from build123d import *

# Parameters (mm, degrees)
EXTRUDE_THIN1_DEPTH             = 57.15
M2_5_CLEARANCE_HOLE1_AT_2_COUNT = 2
M2_5_CLEARANCE_HOLE1_AT_2_PITCH = 6.096
CUT_EXTRUDE1_REACH              = 141.7
SKETCH2_R                       = 6.35
CIRPATTERN1_COUNT               = 8
CUT_EXTRUDE2_REACH              = 59.15
SKETCH5_R                       = 3.5
CIRPATTERN2_COUNT               = 4


with BuildPart() as part:
    # Sketch1 → Extrude-Thin1 (new body)
    with BuildSketch(Plane(origin=(0, 0, 0), x_dir=(0, 0, -1), z_dir=(1, 0, 0))):
        Polygon((0, 0), (57.15, 0), (57.15, -139.7), (52.324, -139.7), (52.324, -4.826), (0, -4.826), align=None)
    extrude(amount=EXTRUDE_THIN1_DEPTH)

    # Sketch4 → M2.5 Clearance Hole1 (revolve, cut)
    with BuildSketch(Plane(origin=(17.349679849, 0, -39.800320151), x_dir=(0, 0, 1), z_dir=(1, 0, 0))):
        Polygon((0, 0), (0, 5.89269403), (1.35255, 5.08), (1.35255, 0), align=None)
    m2_5_clearance_hole1 = revolve(axis=Axis((17.349679849, 6.35, -39.800320151), (0, -1, 0)), mode=Mode.SUBTRACT)

    # M2.5 Clearance Hole1 at 2: M2.5 Clearance Hole1 ×2
    with Locations(*[Vector(0.707106781, 0, 0.707106781) * (i * M2_5_CLEARANCE_HOLE1_AT_2_PITCH) for i in range(1, M2_5_CLEARANCE_HOLE1_AT_2_COUNT)]):
        add(m2_5_clearance_hole1, mode=Mode.SUBTRACT)

    # Sketch2 → Cut-Extrude1 (cut, up to next)
    with BuildSketch(Plane(origin=(0, 0, 0), x_dir=(1, 0, 0), z_dir=(0, 1, 0)), mode=Mode.PRIVATE) as cut_extrude1_sk1:
        with Locations((28.575, 28.575)):
            Circle(SKETCH2_R)
    cut_extrude1_tool1 = extrude(cut_extrude1_sk1.sketch, amount=-CUT_EXTRUDE1_REACH, mode=Mode.PRIVATE) & part.part
    add(cut_extrude1_tool1.solids().sort_by_distance((28.575, 0, -28.575))[0], mode=Mode.SUBTRACT)

    # CirPattern1: M2.5 Clearance Hole1 ×8 about axis
    cirpattern1_axis = Axis((28.575, 0, -28.575), (0, 1, 0))
    for i in range(1, CIRPATTERN1_COUNT):
        add(m2_5_clearance_hole1.rotate(cirpattern1_axis, i * 360 / CIRPATTERN1_COUNT), mode=Mode.SUBTRACT)

    # CirPattern1 copy 1 sketch → CirPattern1 copy 1 (revolve, cut)
    with BuildSketch(Plane(origin=(18.796, 0, -28.575), x_dir=(0.707106781, 0, 0.707106781), z_dir=(0.707106781, 0, -0.707106781))):
        Polygon((0, 0), (0, 5.89269403), (1.35255, 5.08), (1.35255, 0), align=None)
    revolve(axis=Axis((18.796, 6.35, -28.575), (0, -1, 0)), mode=Mode.SUBTRACT)

    # CirPattern1 copy 2 sketch → CirPattern1 copy 2 (revolve, cut)
    with BuildSketch(Plane(origin=(21.660202787, 0, -21.660202787), x_dir=(1, 0, 0), z_dir=(0, 0, -1))):
        Polygon((0, 0), (0, 5.89269403), (1.35255, 5.08), (1.35255, 0), align=None)
    revolve(axis=Axis((21.660202787, 6.35, -21.660202787), (0, -1, 0)), mode=Mode.SUBTRACT)

    # CirPattern1 copy 3 sketch → CirPattern1 copy 3 (revolve, cut)
    with BuildSketch(Plane(origin=(28.575, 0, -18.796), x_dir=(0.707106781, 0, -0.707106781), z_dir=(-0.707106781, 0, -0.707106781))):
        Polygon((0, 0), (0, 5.89269403), (1.35255, 5.08), (1.35255, 0), align=None)
    revolve(axis=Axis((28.575, 6.35, -18.796), (0, -1, 0)), mode=Mode.SUBTRACT)

    # CirPattern1 copy 4 sketch → CirPattern1 copy 4 (revolve, cut)
    with BuildSketch(Plane(origin=(35.489797213, 0, -21.660202787), x_dir=(0, 0, -1), z_dir=(-1, 0, 0))):
        Polygon((0, 0), (0, 5.89269403), (1.35255, 5.08), (1.35255, 0), align=None)
    revolve(axis=Axis((35.489797213, 6.35, -21.660202787), (0, -1, 0)), mode=Mode.SUBTRACT)

    # CirPattern1 copy 5 sketch → CirPattern1 copy 5 (revolve, cut)
    with BuildSketch(Plane(origin=(38.354, 0, -28.575), x_dir=(-0.707106781, 0, -0.707106781), z_dir=(-0.707106781, 0, 0.707106781))):
        Polygon((0, 0), (0, 5.89269403), (1.35255, 5.08), (1.35255, 0), align=None)
    revolve(axis=Axis((38.354, 6.35, -28.575), (0, -1, 0)), mode=Mode.SUBTRACT)

    # CirPattern1 copy 6 sketch → CirPattern1 copy 6 (revolve, cut)
    with BuildSketch(Plane(origin=(35.489797213, 0, -35.489797213), x_dir=(-1, 0, 0), z_dir=(0, 0, 1))):
        Polygon((0, 0), (0, 5.89269403), (1.35255, 5.08), (1.35255, 0), align=None)
    revolve(axis=Axis((35.489797213, 6.35, -35.489797213), (0, -1, 0)), mode=Mode.SUBTRACT)

    # CirPattern1 copy 7 sketch → CirPattern1 copy 7 (revolve, cut)
    with BuildSketch(Plane(origin=(28.575, 0, -38.354), x_dir=(-0.707106781, 0, 0.707106781), z_dir=(0.707106781, 0, 0.707106781))):
        Polygon((0, 0), (0, 5.89269403), (1.35255, 5.08), (1.35255, 0), align=None)
    revolve(axis=Axis((28.575, 6.35, -38.354), (0, -1, 0)), mode=Mode.SUBTRACT)

    # Sketch5 → Cut-Extrude2 (cut, up to next)
    with BuildSketch(Plane(origin=(0, 0, -57.15), x_dir=(-1, 0, 0), z_dir=(0, 0, -1)), mode=Mode.PRIVATE) as cut_extrude2_sk1:
        with Locations((-28.575, -120.65)):
            Circle(SKETCH5_R)
    cut_extrude2_tool1 = extrude(cut_extrude2_sk1.sketch, amount=-CUT_EXTRUDE2_REACH, mode=Mode.PRIVATE) & part.part
    add(cut_extrude2_tool1.solids().sort_by_distance((28.575, -120.65, -57.15))[0], mode=Mode.SUBTRACT)

    # Sketch7 → M3 Clearance Hole1 (revolve, cut)
    with BuildSketch(Plane(origin=(28.575, -107.65, -57.15), x_dir=(0, 1, 0), z_dir=(1, 0, 0))):
        Polygon((0, 0), (0, 6.04137699), (1.6, 5.08), (1.6, 0), align=None)
    m3_clearance_hole1 = revolve(axis=Axis((28.575, -107.65, -63.5), (0, 0, 1)), mode=Mode.SUBTRACT)

    # CirPattern2: M3 Clearance Hole1 ×4 about axis
    cirpattern2_axis = Axis((28.575, -120.65, 0), (0, 0, 1))
    for i in range(1, CIRPATTERN2_COUNT):
        add(m3_clearance_hole1.rotate(cirpattern2_axis, i * 360 / CIRPATTERN2_COUNT), mode=Mode.SUBTRACT)


solid = part.part
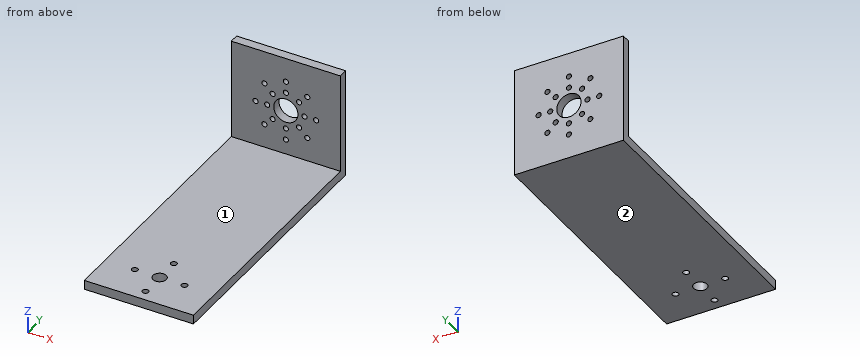
Input: part model. Units: mm. Frame: model coordinates. Face numbers are marked on the shaded views. A direction names the side the tool comes from. Round coordinates to 2 decimals unless told otherwise and drop trailing zeros. Order: outer loops, then holes, each group sorted by start corner. A loop starts at its lowest first (then second) coordinate and runs counter-clockwise, first axis right, second up.
1. Set-up query: the marked faces 1 and 2. Return all of +Z, -Z, +X, -X, +Y, -Y with unobstructed straight access to the full face (end or side cutting, diameter ignored); none if empty.
The answers:
face 1: +Z, +X, -X, -Y
face 2: -Z, +X, -X, +Y, -Y
2. Cut plane A-A, the plane y = -120.65. Output: boundary loops of the cut face in (x, z) (3 decimals).
The answers:
outline: (0, -57.15) - (13.975, -57.15) - (13.975, -52.324) - (0, -52.324) - close; (17.175, -57.15) - (25.075, -57.15) - (25.075, -52.324) - (17.175, -52.324) - close; (32.075, -57.15) - (39.975, -57.15) - (39.975, -52.324) - (32.075, -52.324) - close; (43.175, -57.15) - (57.15, -57.15) - (57.15, -52.324) - (43.175, -52.324) - close
3. Cut plane B-B, the plane x = 5. Output: boundary loops of the cut face in (y, z).
The answers:
outline: (-139.7, -57.15) - (0, -57.15) - (0, 0) - (-4.83, 0) - (-4.83, -52.32) - (-139.7, -52.32) - close
4. Cut plane D-D, the plane z = -4.5. Output: boundary loops of the cut face in (x, y), then the cut area to 3 significant figures.
The answers:
outline: (0, -4.83) - (57.15, -4.83) - (57.15, 0) - (0, 0) - close
area: 276 mm2
5. Pin query (flat end, axial travel): P1, Ø2, axis at x = 28.575, z = -18.796, coming from the -Y side; P2, Ø1, axis at x = 16, y = -15, coming from the +Z side; P3, Ø12, axis at x = 15.5, z = -25, coming from the -Y side. Return the tip coordinate at first contact, or that it passes through.
The answers:
P1: passes through
P2: stops at z = -52.32
P3: stops at y = -4.83
6. Cut plane C-C, the plane y = -38. Output: boundary loops of the cut face in (x, z), then the cut area to 3 significant figures.
The answers:
outline: (0, -57.15) - (57.15, -57.15) - (57.15, -52.32) - (0, -52.32) - close
area: 276 mm2
7. Material intervals for line 1 (Z direction, x = 43.5, y = -117.5); line 2 (Y direction, x = 11.5, z = -19); line 3 (Y direction, x = 16, z = -52.5), sorted ascending.
The answers:
line 1: z = -57.15 to -52.32
line 2: y = -4.83 to 0
line 3: y = -139.7 to -122.19, -119.11 to 0
